Part print with two shaded views. Sizes in mm from the minimum x, y, z corner. A direction names the side the tool comes from. Round coordinates to 2 decimals unless told otherwise and drop trailing zeros. Loops run counter-clockwise (first coordinate to the right, second up) from the corner with the lowest first, then second, coordinate; pieces in that order, holes last. Notation, with made-up numbers: (-37.5, 51.5) - (-15.5, 51.5) arc R14 ccw to (-15.5, 71.5) - close; hole circle Ø9 at (84, 61.5). An arc over 180 degrees is marked (long way). One line per question, with ' | ' between items.
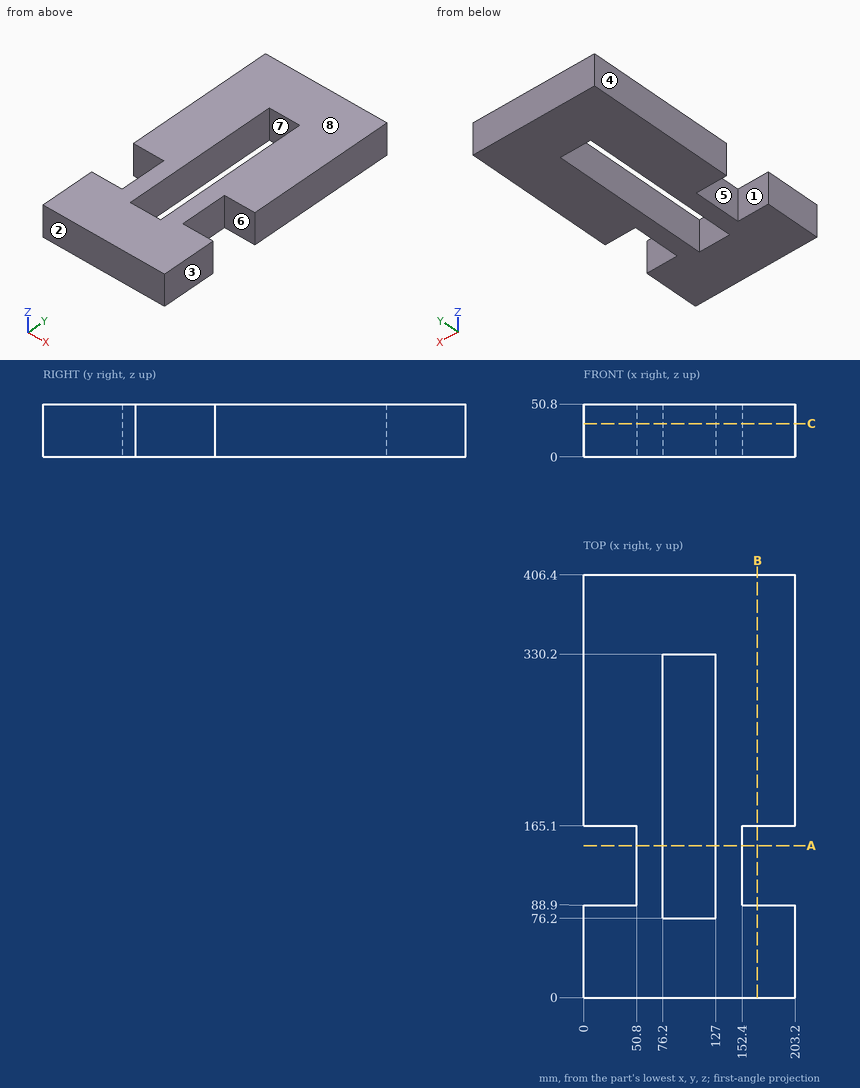
(1) Tool access for the marked faces 4, 5, 6, 7 and 8: list every direction of +Z, -Z, +X, -X, +Y, -Y with a clear straight run to the whole face (end or side of a thin tool).
Results found:
face 4: +Z, -Z, -X, +Y, -Y | face 5: +Z, -Z, -X | face 6: +Z, -Z, +X | face 7: +Z, -Z | face 8: +Z, +X, -X, +Y, -Y
(2) Cut at A-A, the plane y = 146. Write the cut outline in (x, z), then the cut area to 3 significant figures.
Results found:
outline: (50.8, 0) - (76.2, 0) - (76.2, 50.8) - (50.8, 50.8) - close; (127, 0) - (152.4, 0) - (152.4, 50.8) - (127, 50.8) - close | area: 2,580 mm²
(3) Two-plate mould, pull along Y, no slides. Class the marked faces 1, 2 and 3: released by +Y, released by -Y, zero draft, split by the parting line, or undercut.
Results found:
face 1: undercut | face 2: released by -Y | face 3: zero draft
(4) Cut at B-B, the plane x = 167. Write the cut outline in (y, z), then the cut area to 3 significant figures.
Results found:
outline: (0, 0) - (88.9, 0) - (88.9, 50.8) - (0, 50.8) - close; (165.1, 0) - (406.4, 0) - (406.4, 50.8) - (165.1, 50.8) - close | area: 16,800 mm²
(5) Cut at C-C, the plane z = 32. Write the cut outline in (x, y), then the cut area to 3 significant figures.
Results found:
outline: (0, 0) - (203.2, 0) - (203.2, 88.9) - (152.4, 88.9) - (152.4, 165.1) - (203.2, 165.1) - (203.2, 406.4) - (0, 406.4) - (0, 165.1) - (50.8, 165.1) - (50.8, 88.9) - (0, 88.9) - close; hole (76.2, 76.2) - (127, 76.2) - (127, 330.2) - (76.2, 330.2) - close | area: 61,900 mm²
(6) Probe L1, parallel to X at y = 315, z = 17.5; L2, parallel to X at y = 159.5, z = 9.5; L3, parallel to Y at x = 95.5, z = 42. List the from-to ranges inside material, lowest first.
Results found:
L1: x = 0 to 76.2, 127 to 203.2 | L2: x = 50.8 to 76.2, 127 to 152.4 | L3: y = 0 to 76.2, 330.2 to 406.4
